Here's how the part is built. I have some questions about the finished solid (model axes, mm). A direction names the side the tool comes from. Coordinates: 2 decimals unless noted, no trailing zeros. Write each loop counter-clockwise with the first axis right and the second up, starting at its lowest first coordinate (ties: lowest second). Pieces come first, ordered by that corner, then holes. Notation, with made-up numbers: (88.5, 25) -> (103.5, 25) arc R29 cw to (103.5, 63) -> close; hole circle Ø11 at (21.25, -19.5). An arc over 180 degrees is marked (long way). Use a Markdown table: item, result. Add a question column.
Item 1: Imagine slicing it at D-D, the plane x = 0. Write out the boundary of the cut face in (y, z), and give its area (3 significant figures).
Item 2: If I drill on line 1 along Z through (x, y) = (0, -2.5); line 2 along X through (y, z) = (-1.7, 2.25); line 3 along X through (y, z) = (-2.4, 5), over which ranges is the centre line in solid material (lowest first)? Write a range as from..to.
Item 3: Imagine slicing it at A-A, the plane x = 1.75. Write out the boundary of the cut face in (y, z), and give its area (3 significant figures).
Item 4: Imagine slicing it at B-B, the plane z = -6.5. Write out the boundary of the cut face in (x, y).
Item 5: If we mould it in two halves opening along X, with no side actions, what happens to faces 4 (the flat face through (-3.75, 0.5, 2.1)), 5 (the flat face through (2, -2.5, -6.5)), 6 (the cylindrical face through (0.13, -2.51, 4.01)), 7 (the flat face through (0, 0, 2))? For each: pulls with the +X half, pulls with the -X half, needs draft (parallel to the pull), parting line crosses it, or undercut.
Item 6: Will these pins go through, and if not, where does the flat tip stop? pin 1 Ø4 at (x, z) = (-4.5, 0.5) entering from +Y; pin 2 Ø0.7 at (x, y) = (-3.5, 1.5) entering from -Z; pin 3 Ø0.5 at (y, z) = (0.5, -6) entering from +X; pin 4 Ø3 at (x, z) = (0, -5) entering from -Y.
Item 7: Imagine slicing it at C-C, the plane y = -2.6. Write out the boundary of the cut face in (x, z).
Item 8: On a 3-axis mill with a long thin cutter (end or side, diameter ignored), from which of +Z, -Z, +X, -X, +Y, -Y can I reach the whole of each face in a straight line? I mean faces 1 (the flat face through (4, -2, -1)), 2 (the flat face through (-4, -2, -2)), 3 (the flat face through (-1.5, 0.5, -6.7)). Say none if no direction works.
```python
from build123d import *

# Parameters (mm, degrees)
SKETCH1_W            = 7.5
SKETCH1_H            = 10
BOSS_EXTRUDE1_DEPTH  = 1
SKETCH10_W           = 7.5
SKETCH10_H           = 1
BOSS_EXTRUDE5_DEPTH  = 2
SKETCH56_W           = 7.5
SKETCH56_H           = 1
BOSS_EXTRUDE17_DEPTH = 2
SKETCH57_W           = 3
SKETCH57_H           = 1
BOSS_EXTRUDE18_DEPTH = 5
SKETCH58_W           = 1.5
SKETCH58_H           = 1
BOSS_EXTRUDE19_DEPTH = 2
SKETCH59_W           = 1.5
SKETCH59_H           = 1
BOSS_EXTRUDE20_DEPTH = 2
SKETCH60_W           = 1
SKETCH60_H           = 1.5
BOSS_EXTRUDE23_DEPTH = 1.5
SKETCH61_W           = 1
SKETCH61_H           = 0.75
CUT_EXTRUDE1_DEPTH   = 0.5
SKETCH62_W           = 6
SKETCH62_H           = 12
BOSS_EXTRUDE25_DEPTH = 3
SKETCH64_W           = 4
SKETCH64_H           = 2
CUT_EXTRUDE2_DEPTH   = 12
SKETCH65_W           = 4
SKETCH65_H           = 1
BOSS_EXTRUDE26_DEPTH = 3
SKETCH66_R           = 1
CUT_EXTRUDE3_DEPTH   = 1
SKETCH69_W           = 7
SKETCH69_H           = 1.5
CUT_EXTRUDE8_DEPTH   = 10
SKETCH70_W           = 0.6
SKETCH70_H           = 1.8
BOSS_EXTRUDE27_DEPTH = 1
SKETCH68_W           = 3
SKETCH68_H           = 1
BOSS_EXTRUDE28_DEPTH = 3
SKETCH67_W           = 3
SKETCH67_H           = 1
BOSS_EXTRUDE29_DEPTH = 3


with BuildPart() as part:
    # Sketch1 → Boss-Extrude1 (new body)
    with BuildSketch(Plane(origin=(0, 0, 0), x_dir=(1, 0, 0), z_dir=(0, 1, 0))):
        Rectangle(SKETCH1_W, SKETCH1_H)
    extrude(amount=BOSS_EXTRUDE1_DEPTH)

    # Sketch10 → Boss-Extrude5 (add)
    with BuildSketch(Plane.XY.offset(5)):
        with Locations((0, 0.5)):
            Rectangle(SKETCH10_W, SKETCH10_H)
    extrude(amount=BOSS_EXTRUDE5_DEPTH)

    # Sketch56 → Boss-Extrude17 (add)
    with BuildSketch(Plane.XY.offset(7)):
        with Locations((0, 0.5)):
            Rectangle(SKETCH56_W, SKETCH56_H)
    extrude(amount=BOSS_EXTRUDE17_DEPTH)

    # Sketch57 → Boss-Extrude18 (add)
    with BuildSketch(Plane(origin=(0, 0, -5), x_dir=(-1, 0, 0), z_dir=(0, 0, -1))):
        with Locations((0, 0.5)):
            Rectangle(SKETCH57_W, SKETCH57_H)
    extrude(amount=BOSS_EXTRUDE18_DEPTH)

    # Sketch58 → Boss-Extrude19 (add)
    with BuildSketch(Plane(origin=(1.5, 0, 0), x_dir=(0, 0, -1), z_dir=(1, 0, 0))):
        with Locations((9.25, 0.5)):
            Rectangle(SKETCH58_W, SKETCH58_H)
    extrude(amount=BOSS_EXTRUDE19_DEPTH)

    # Sketch59 → Boss-Extrude20 (add)
    with BuildSketch(Plane.ZY.offset(1.5)):
        with Locations((-9.25, 0.5)):
            Rectangle(SKETCH59_W, SKETCH59_H)
    extrude(amount=BOSS_EXTRUDE20_DEPTH)

    # Sketch60 → Boss-Extrude23 (add)
    with BuildSketch(Plane(origin=(0, 1, 0), x_dir=(1, 0, 0), z_dir=(0, 1, 0))):
        with Locations((3, 9.25)):
            Rectangle(SKETCH60_W, SKETCH60_H)
        with Locations((-3, 9.25)):
            Rectangle(SKETCH60_W, SKETCH60_H)
    extrude(amount=BOSS_EXTRUDE23_DEPTH)

    # Sketch61 → Cut-Extrude1 (cut)
    with BuildSketch(Plane(origin=(0, 2.5, 0), x_dir=(1, 0, 0), z_dir=(0, 1, 0))):
        with Locations((-3, 9.245443114)):
            Rectangle(SKETCH61_W, SKETCH61_H)
        with Locations((3, 9.245443114)):
            Rectangle(SKETCH61_W, SKETCH61_H)
    extrude(amount=-CUT_EXTRUDE1_DEPTH, mode=Mode.SUBTRACT)

    # Sketch62 → Boss-Extrude25 (add)
    with BuildSketch(Plane(origin=(0, 0, 0), x_dir=(-1, 0, 0), z_dir=(0, -1, 0))):
        with Locations((0, -1)):
            Rectangle(SKETCH62_W, SKETCH62_H)
    extrude(amount=BOSS_EXTRUDE25_DEPTH)

    # Sketch64 → Cut-Extrude2 (cut)
    with BuildSketch(Plane.XY.offset(7)):
        with Locations((0, -1)):
            Rectangle(SKETCH64_W, SKETCH64_H)
    extrude(amount=-CUT_EXTRUDE2_DEPTH, mode=Mode.SUBTRACT)

    # Sketch65 → Boss-Extrude26 (add)
    with BuildSketch(Plane(origin=(0, 0, -5), x_dir=(-1, 0, 0), z_dir=(0, 0, -1))):
        with Locations((0, -2.5)):
            Rectangle(SKETCH65_W, SKETCH65_H)
    extrude(amount=BOSS_EXTRUDE26_DEPTH)

    # Sketch66 → Cut-Extrude3 (cut)
    with BuildSketch(Plane(origin=(0, -3, 0), x_dir=(-1, 0, 0), z_dir=(0, -1, 0))):
        with Locations((0, -5)):
            Circle(SKETCH66_R)
        with Locations((0, 5)):
            Circle(SKETCH66_R)
    extrude(amount=-CUT_EXTRUDE3_DEPTH, mode=Mode.SUBTRACT)

    # Sketch69 → Cut-Extrude8 (cut)
    with BuildSketch(Plane.XZ):
        with Locations((0, -9.25)):
            Rectangle(SKETCH69_W, SKETCH69_H)
    extrude(amount=-CUT_EXTRUDE8_DEPTH, mode=Mode.SUBTRACT)

    # Sketch70 → Boss-Extrude27 (add)
    with BuildSketch(Plane(origin=(0, 1, 0), x_dir=(1, 0, 0), z_dir=(0, 1, 0))):
        with Locations((-3.45, -8.1)):
            Rectangle(SKETCH70_W, SKETCH70_H)
        with Locations((3.45, -8.1)):
            Rectangle(SKETCH70_W, SKETCH70_H)
    extrude(amount=BOSS_EXTRUDE27_DEPTH)

    # Sketch68 → Boss-Extrude28 (add)
    with BuildSketch(Plane(origin=(3, 0, 0), x_dir=(0, 0, -1), z_dir=(1, 0, 0))):
        with Locations((1.5, -1.5)):
            Rectangle(SKETCH68_W, SKETCH68_H)
    extrude(amount=BOSS_EXTRUDE28_DEPTH)

    # Sketch67 → Boss-Extrude29 (add)
    with BuildSketch(Plane.ZY.offset(3)):
        with Locations((-1.5, -1.5)):
            Rectangle(SKETCH67_W, SKETCH67_H)
    extrude(amount=BOSS_EXTRUDE29_DEPTH)


solid = part.part
```
Ans:
| question | item | result |
|---|---|---|
| 1 | outline | (-3, -8) -> (-2, -8) -> (-2, -6) -> (-3, -6) -> close; (-3, -4) -> (-2, -4) -> (-2, 4) -> (-3, 4) -> close; (-3, 6) -> (-2, 6) -> (-2, 7) -> (-3, 7) -> close; (0, -8.5) -> (1, -8.5) -> (1, 9) -> (0, 9) -> close |
| 1 | area | 28.5 mm^2 |
| 2 | line 1 | z = -8..-6, -4..4, 6..7 |
| 2 | line 2 | x = -3..-2, 2..3 |
| 2 | line 3 | x = -3..-1, 1..3 |
| 3 | outline | (-3, -8) -> (-2, -8) -> (-2, 7) -> (-3, 7) -> close; (0, -5) -> (1, -5) -> (1, 9) -> (0, 9) -> close |
| 3 | area | 29.0 mm^2 |
| 4 | outline | (-2, -3) -> (2, -3) -> (2, -2) -> (-2, -2) -> close; (-1.5, 0) -> (1.5, 0) -> (1.5, 1) -> (-1.5, 1) -> close |
| 5 | face 4 | pulls with the -X half |
| 5 | face 5 | pulls with the +X half |
| 5 | face 6 | undercut |
| 5 | face 7 | undercut |
| 6 | pin 1 | stops at y = 1 |
| 6 | pin 2 | stops at z = 7.2 |
| 6 | pin 3 | stops at x = 1.5 |
| 6 | pin 4 | stops at y = -3 |
| 7 | outline | (-3, -5) -> (-2, -5) -> (-2, -8) -> (2, -8) -> (2, -5) -> (3, -5) -> (3, 7) -> (-3, 7) -> close; hole circle Ø2 at (0, -5); hole circle Ø2 at (0, 5) |
| 8 | face 1 | +Z, -Z, +X, -Y |
| 8 | face 2 | +Z, -Z, -X, -Y |
| 8 | face 3 | -Z, -X, +Y |
